```python
from build123d import *

# Parameters (mm, degrees)
SKETCH1_RX               = 20
SKETCH1_RY               = 10
BOSS_EXTRUDE1_DEPTH      = 2
BOSS_EXTRUDE2_DEPTH      = 1.5
BOSS_EXTRUDE2_DEPTH_BACK = 1.5
SKETCH2_W                = 5
SKETCH2_H                = 2
SKETCH3_W                = 4.15
SKETCH3_H                = 1.5
BOSS_EXTRUDE3_DEPTH      = 10
FILLET1_R                = 1
FILLET3_R                = 0.5


with BuildPart() as part:
    # Sketch1 → Boss-Extrude1 (new body)
    with BuildSketch(Plane.XY):
        with Locations((0, 0)):
            Ellipse(SKETCH1_RX, SKETCH1_RY)
    extrude(amount=BOSS_EXTRUDE1_DEPTH)

    # Sketch2 → Boss-Extrude2 (add, two sides: drawn at the far end of the back side and taken through both)
    with BuildSketch(Plane(origin=(0, 0, 0), x_dir=(1, 0, 0), z_dir=(0, 1, 0)).offset(-BOSS_EXTRUDE2_DEPTH_BACK)):
        with Locations((0, -3)):
            Rectangle(SKETCH2_W, SKETCH2_H)
    extrude(amount=BOSS_EXTRUDE2_DEPTH + BOSS_EXTRUDE2_DEPTH_BACK)

    # Sketch3 → Boss-Extrude3 (add)
    with BuildSketch(Plane.XY.offset(4)):
        Rectangle(SKETCH3_W, SKETCH3_H)
    extrude(amount=BOSS_EXTRUDE3_DEPTH)

    # Fillet1
    fillet1_edges = [part.edges().sort_by_distance(p)[0] for p in [
        (-2.5, -1.5, 3),
        (2.5, -1.5, 3),
        (-2.5, 1.5, 3),
        (2.5, 1.5, 3),
    ]]
    fillet(fillet1_edges, radius=FILLET1_R)

    # Fillet3
    fillet3_edges = [part.edges().sort_by_distance(p)[0] for p in [
        (-2.075, 0.75, 9),
        (-2.075, -0.75, 9),
        (2.075, -0.75, 9),
        (2.075, 0.75, 9),
        (-2.075, 0, 14),
        (0, -0.75, 14),
        (2.075, 0, 14),
        (0, 0.75, 14),
    ]]
    fillet(fillet3_edges, radius=FILLET3_R)


solid = part.part
```
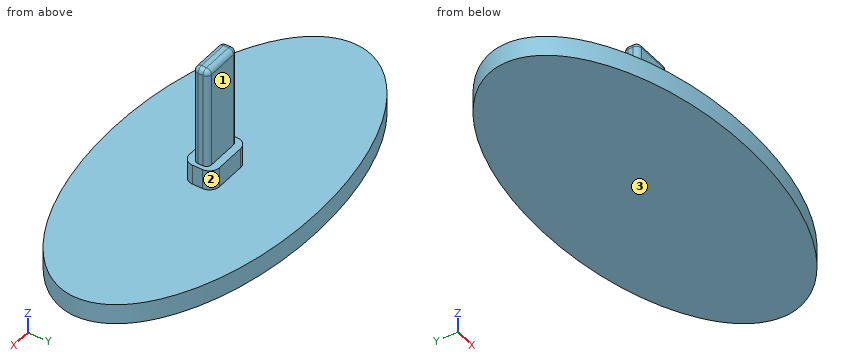
Input: part model. Units: mm. Frame: model coordinates. Face numbers are marked on the shaded views. A direction names the side the tool comes from. Round coordinates to 2 decimals unless told otherwise and drop trailing zeros. Loops run counter-clockwise (first coordinate to the right, second up) from the corner with the lowest first, then second, coordinate; pieces in that order, holes last.
1) Material intervals for line 1 (Z direction, x = -18, y = -0.75); line 2 (Y direction, x = 0, z = 10); line 3 (Y direction, x = 2, z = 7.5), sorted ascending.
Ans:
line 1: z = 0 to 2
line 2: y = -0.75 to 0.75
line 3: y = -0.51 to 0.51
2) Section query B-B on z = 10.75. Return the cut outline in (x, y) (3 decimals).
Ans:
outline: (-2.075, -0.25) arc R0.5 ccw to (-1.575, -0.75) - (1.575, -0.75) arc R0.5 ccw to (2.075, -0.25) - (2.075, 0.25) arc R0.5 ccw to (1.575, 0.75) - (-1.575, 0.75) arc R0.5 ccw to (-2.075, 0.25) - close
3) Set-up query: the marked faces 1, 2 and 3. Return all of +Z, -Z, +X, -X, +Y, -Y with unobstructed straight access to the full face (end or side cutting, diameter ignored); none if empty.
Ans:
face 1: +Z, +X, -X, +Y
face 2: +Z, +X, +Y
face 3: -Z, +X, -X, +Y, -Y
4) Section query A-A on z = 3. Return the cut outline in (x, y), plus the area to 3 significant figures.
Ans:
outline: (-2.5, -0.5) arc R1 ccw to (-1.5, -1.5) - (1.5, -1.5) arc R1 ccw to (2.5, -0.5) - (2.5, 0.5) arc R1 ccw to (1.5, 1.5) - (-1.5, 1.5) arc R1 ccw to (-2.5, 0.5) - close
area: 14.1 mm2
5) Pin query (flat end, axial travel): pin 1 (0.6 mm diameter, centred on y = 0, z = 8, fed in from -X) (3 decimals); pin 2 (0.9 mm diameter, centred on x = 0.5, z = 10.5, fed in from +Y); pin 3 (8 mm diameter, centred on x = 7.5, z = 11.5, fed in from -Y); pin 4 (6 mm diameter, centred on x = -5, y = -4, fed in from +Z). Return the tip coordinate at first contact, or that it passes through.
Ans:
pin 1: stops at x = -2.075
pin 2: stops at y = 0.75
pin 3: passes through
pin 4: stops at z = 2
